Part model, mm, in its own coordinate system. Give positions to 0.01 mm unless a question says otherwise; leave off trailing zeros. Order: outer loops, then holes, each group sorted by start corner. A loop starts at its lowest first (then second) coordinate and runs counter-clockwise, first axis right, second up. Notation, with made-up numbers: (64, 69) - (83, 69) arc R13 cw to (83, 92) - close; hole circle Ø6 at (-15.5, 32.25). An arc over 180 degrees is marked (long way). One line per item, written item: value.
```python
from build123d import *

# Parameters (mm, degrees)
CORTAR_EXTRUIR3_DEPTH = 45
CROQUIS6_R            = 1.65
CORTAR_EXTRUIR4_DEPTH = 20


with BuildPart() as part:
    # Croquis1 → Revolución3 (revolve)
    with BuildSketch(Plane(origin=(0, 0, 0), x_dir=(1, 0, 0), z_dir=(0, 1, 0))):
        with BuildLine():
            Line((-12.5, 0), (-20.5, 0))
            Line((-20.5, 0), (-20.5, 14.049477092))
            Line((-20.5, 14.049477092), (9.52106407, 14.049477092))
            Line((9.52106407, 14.049477092), (9.399951047, 8.239594669))
            ThreePointArc((9.399951047, 8.239594669), (-4.40173897, 11.699345881), (-12.5, 0))
        make_face()
    revolve(axis=Axis((-12.5, 0, 0), (-1, 0, 0)))

    # Croquis5 → Cortar-Extruir3 (cut)
    with BuildSketch(Plane.ZY.offset(20.5)):
        Polygon((0, 0), (-16.832618664, 0), (-16.832618664, 15.474654251), (15.925083383, 15.474654251), (15.925083383, 0), align=None)
    extrude(amount=-CORTAR_EXTRUIR3_DEPTH, mode=Mode.SUBTRACT)

    # Croquis6 → Cortar-Extruir4 (cut)
    with BuildSketch(Plane(origin=(0, 0, 0), x_dir=(1, 0, 0), z_dir=(0, 1, 0))):
        with Locations((-17.221724739, 0)):
            Circle(CROQUIS6_R)
    extrude(amount=-CORTAR_EXTRUIR4_DEPTH, mode=Mode.SUBTRACT)


solid = part.part
```
1) Cut at A-A, the plane z = 0. Give the cut face in (x, y).
Outcome:
outline: (-20.5, -14.05) - (-18.87, -14.05) - (-18.87, 0) - (-20.5, 0) - close; (-15.57, -14.05) - (9.52, -14.05) - (9.4, -8.24) arc R12.5 cw to (-12.5, 0) - (-15.57, 0) - close
2) Drill centre lines: line 1 along X through (y, z) = (-7, 5.5); line 2 along Z through (x, y) = (3.5, -0.75); line 3 along X through (y, z) = (-10, 4.75). Where is each one in solid material? Low to high. Write a range as from..to.
Outcome:
line 1: x = -20.5..-8.77, 8.77..9.41
line 2: z = -14.03..-11.98, 11.98..14.03
line 3: x = -20.5..-5.8, 5.8..9.46
3) Pin check, flat tips, straight feed: pin 1 (4 mm diameter, centred on x = -1.5, y = -12, fed in from -Z); pin 2 (8 mm diameter, centred on y = -5, z = 4.5, fed in from +X); pin 3 (3 mm diameter, centred on x = -16, z = -5.5, fed in from -Y); pin 4 (6 mm diameter, centred on x = -5.5, z = -2, fed in from -Y). Stop position of each tip, or through.
Outcome:
pin 1: stops at z = -9.87
pin 2: stops at x = 9.45
pin 3: stops at y = -13.47
pin 4: stops at y = -14.05
4) Mould opens along Z. For faces 1 (the flat face through (-20.5, -6, 0)), 2 (the cylindrical face through (-15.698, -6.928, 0.632)), 3 (the conical face through (9.406, -8.52, -0.187)), 4 (the cylindrical face through (-5.279, -14.046, -0.309)) say: released by +Z, released by -Z, zero draft, split by the parting line, or undercut.
Outcome:
face 1: zero draft
face 2: undercut
face 3: undercut
face 4: split by the parting line
5) Cut at B-B, the plane x = 0. Give the cut face in (y, z).
Outcome:
outline: (0, -14.05) - (0, -12.5) arc R12.5 cw to (0, 12.5) - (0, 14.05) arc R14.05 ccw to start
6) Cut at D-D, the plane x = -8.5. Give the cut face in (y, z).
Outcome:
outline: (0, -14.05) - (0, -9.17) arc R9.17 cw to (0, 9.17) - (0, 14.05) arc R14.05 ccw to start
7) Cut at C-C, the plane y = -12. Give the number of separate pieces and of enclosed holes in the cut face, then the cut area to 3 significant figures.
Outcome:
separate pieces: 1
enclosed holes: 2
area: 391 mm^2
